Here's the drawing with two shaded views (mm, measured from the low corner). I have some questions. A direction names the side the tool comes from. Round coordinates to 2 decimals unless told otherwise and drop trailing zeros. Loops run counter-clockwise (first coordinate to the right, second up) from the corner with the lowest first, then second, coordinate; pieces in that order, holes last. Notation, with made-up numbers: M -14,15.25 L 31,15.25 A24 ccw 31,48.25 Z; hole C -5,33.5 d8. An arc over 180 degrees is marked long. Answer as a JSON object with one key per item and string values.
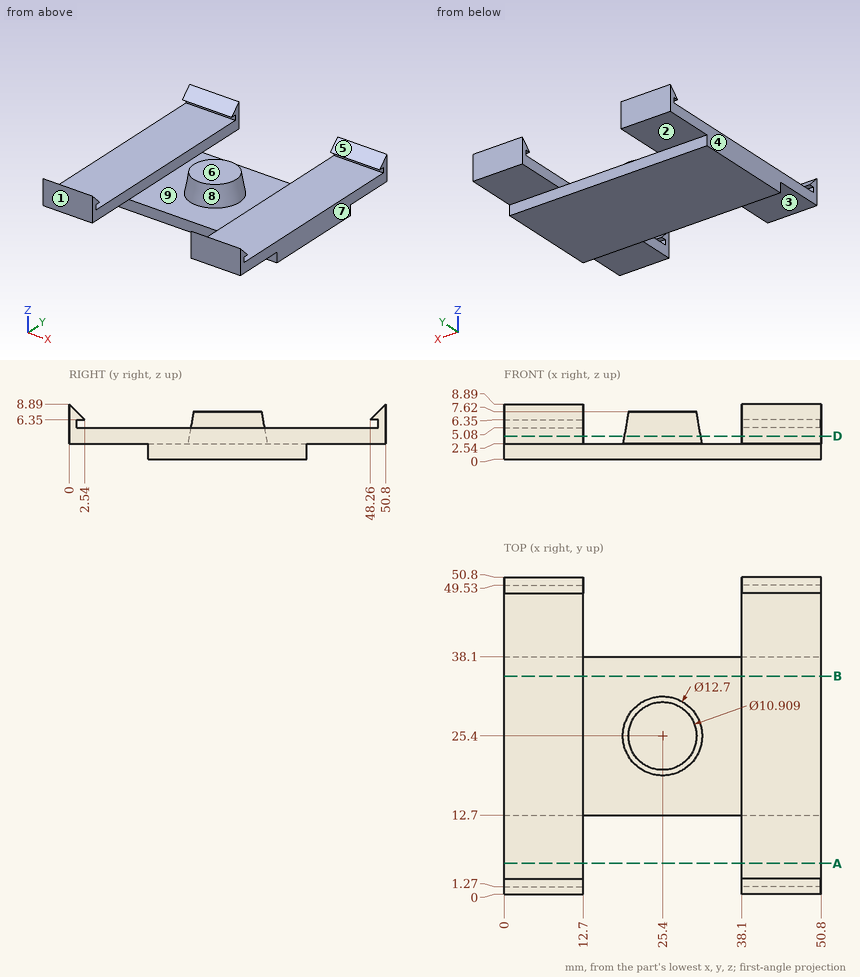
Item 1: If I drill on L1, parallel to X at y = 34.5, z = 4.25; L2, parallel to X at y = 29, z = 5 (1 decimal); L3, parallel to X at y = 26.5, z = 4.5, over which ranges is the centre line in solid material (lowest first)? Write a range as from..to.
Solution:
{"L1": "x = 0..12.7, 38.1..50.8", "L2": "x = 0..12.7, 20.7..30.1, 38.1..50.8", "L3": "x = 0..12.7, 19.5..31.3, 38.1..50.8"}
Item 2: For P1, Ø1.4, axis at x = 6.5, y = 49, coming from the -Z side; P2, Ø3, axis at x = 34.5, z = 2, coming from the -Y side; P3, Ø3, axis at x = 20.5, z = 1, coming from the +Y side, each with a flat end and sliding along its axis, tell me the tip position at first contact or that it passes through.
Solution:
{"P1": "stops at z = 2.54", "P2": "stops at y = 12.7", "P3": "stops at y = 38.1"}
Item 3: I want a section at A-A on y = 5. List the corners of the cut face in (x, z) for me.
Solution:
{"outline": "M 0,2.54 L 12.7,2.54 L 12.7,5.08 L 0,5.08 Z; M 38.1,2.54 L 50.8,2.54 L 50.8,5.08 L 38.1,5.08 Z"}
Item 4: We'd pull the mould along X, two halves only. Please class the marked faces 6, 7, 8 and 9: +X half, -X half, draft (parallel to the pull), parting line (faces both ways), or undercut.
Solution:
{"face 6": "draft", "face 7": "+X half", "face 8": "undercut", "face 9": "undercut"}
Item 5: I want a section at D-D on z = 3.75. List the corners of the cut face in (x, y) for me, plus the area to 3 significant figures.
Solution:
{"outline": "M 0,0 L 12.7,0 L 12.7,50.8 L 0,50.8 Z; C 25.4,25.4 d12.27; M 38.1,0 L 50.8,0 L 50.8,50.8 L 38.1,50.8 Z", "area": "1,410 mm2"}
Item 6: I want a section at B-B on y = 35. List the corners of the cut face in (x, z) for me.
Solution:
{"outline": "M 0,0 L 50.8,0 L 50.8,5.08 L 38.1,5.08 L 38.1,2.54 L 12.7,2.54 L 12.7,5.08 L 0,5.08 Z"}
Item 7: For the marked faces 1, 2, 3, 4 and 5, which set-ups out of +Z, -Z, +X, -X, +Y, -Y let a thin tool reach every point of the face, with its end or its side?
Solution:
{"face 1": "+Z, -Z, +X, -X, -Y", "face 2": "-Z, +X, -X, +Y", "face 3": "-Z, +X, -X, -Y", "face 4": "+Z, -Z, -X, +Y, -Y", "face 5": "+Z, +X, -X"}
